Verification items for this drawing (mm, ordinates from the low corner). A direction names the side the tool comes from. Give positions to 0.01 mm unless a question says otherwise; leave off trailing zeros. Loops run counter-clockwise (first coordinate to the right, second up) from the corner with the lowest first, then second, coordinate; pieces in that order, holes last. Notation, with made-up numbers: M 57.5,-15.5 L 88.5,-15.5 A29 cw 88.5,9.5 Z; hole C 67.25,38.5 d8. An arc over 180 degrees is marked long. Use a Markdown table: item, result.
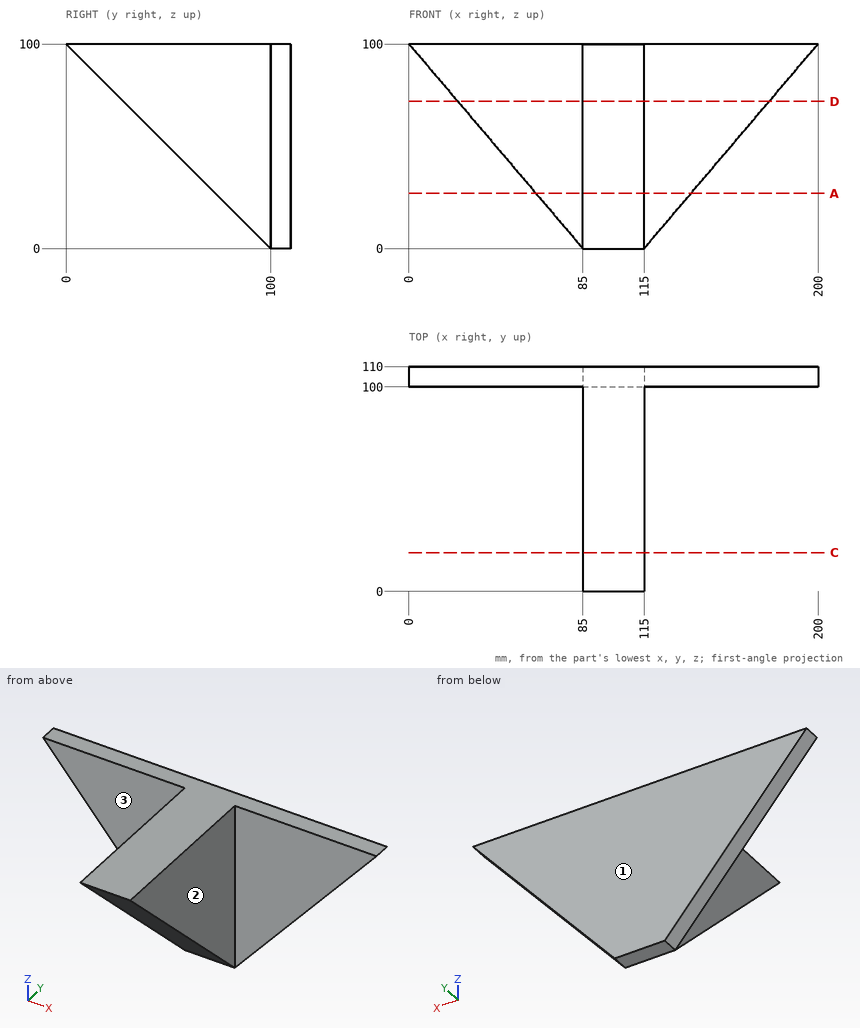
(1) Cross-section at C-C on y = 19. Record the cut outline in (x, z).
Results below:
| item | result |
|---|---|
| outline | M 85,81 L 115,81 L 115,100 L 85,100 Z |
(2) Cross-section at A-A on z = 27. Record the cut outline in (x, y).
Results below:
| item | result |
|---|---|
| outline | M 62.05,100 L 85,100 L 85,73 L 115,73 L 115,100 L 137.95,100 L 137.95,110 L 62.05,110 Z |
(3) Set-up check for the marked faces 1, 2 and 3: record each of +Z, -Z, +X, -X, +Y, -Y from which the full face is reachable in a straight line by a thin tool's end or side.
Results below:
| item | result |
|---|---|
| face 1 | +Z, -Z, +X, -X, +Y |
| face 2 | +Z, -Z, +X, -Y |
| face 3 | +Z, -Z, -X, -Y |
(4) Material ranges on line 1 (X direction, y = 31.5, z = 71); line 2 (Y direction, x = 78, z = 84); line 3 (Y direction, x = 93, z = 85), recorded low to high.
Results below:
| item | result |
|---|---|
| line 1 | 85 to 115 |
| line 2 | 100 to 110 |
| line 3 | 15 to 110 |
(5) Cross-section at D-D on z = 72. Record the cut outline in (x, y).
Results below:
| item | result |
|---|---|
| outline | M 23.8,100 L 85,100 L 85,28 L 115,28 L 115,100 L 176.2,100 L 176.2,110 L 23.8,110 Z |
(6) Gauge pin test, flat ends, axial feed: P1, Ø5, axis at y = 94.5, z = 65.5, coming from the +X side; P2, Ø12, axis at x = 141, z = 85.5, coming from the -Y side. Record the tip position at first contact, or that the pin passes through.
Results below:
| item | result |
|---|---|
| P1 | x = 115 |
| P2 | y = 100 |
